```python
from build123d import *

# Parameters (mm, degrees)
BOSS_EXTRUDE1_DEPTH = 5
SKETCH2_R           = 2.1
SKETCH2_R_2         = 1.5
CUT_EXTRUDE1_DEPTH  = 6
SKETCH4_R           = 2.1
CUT_EXTRUDE2_DEPTH  = 6
FILLET1_R           = 2


with BuildPart() as part:
    # Sketch1 → Boss-Extrude1 (new body)
    with BuildSketch(Plane.XY):
        Polygon((-39, 100.232788632), (-12.5, 134.403841263), (-12.5, 167.075), (12.5, 167.075), (12.5, 134.403841263), (39, 100.232788632), (39, 52.075), (27.012855738, 52.075), (-27.012855738, 52.075), (-39, 52.075), align=None)
    extrude(amount=BOSS_EXTRUDE1_DEPTH)

    # Sketch2 → Cut-Extrude1 (cut, through all)
    with BuildSketch(Plane(origin=(0, 0, 0), x_dir=(-1, 0, 0), z_dir=(0, 0, -1))):
        with Locations((-32, 92.575)):
            Circle(SKETCH2_R)
        with Locations((32, 92.575)):
            Circle(SKETCH2_R)
        with Locations((8, 162.075)):
            Circle(SKETCH2_R)
        with Locations((-8, 162.075)):
            Circle(SKETCH2_R)
        with Locations((-18, 112.575)):
            Circle(SKETCH2_R_2)
    extrude(amount=-CUT_EXTRUDE1_DEPTH, mode=Mode.SUBTRACT)

    # Sketch4 → Cut-Extrude2 (cut, through all)
    with BuildSketch(Plane(origin=(0, 0, 0), x_dir=(-1, 0, 0), z_dir=(0, 0, -1))):
        with Locations((-32, 60.075)):
            Circle(SKETCH4_R)
        with Locations((32, 60.075)):
            Circle(SKETCH4_R)
        with Locations((0, 60.075)):
            Circle(SKETCH4_R)
        with Locations((0, 112.575)):
            Circle(SKETCH4_R)
        with Locations((0, 92.575)):
            Circle(SKETCH4_R)
    extrude(amount=-CUT_EXTRUDE2_DEPTH, mode=Mode.SUBTRACT)

    # Fillet1
    fillet1_edges = [part.edges().sort_by_distance(p)[0] for p in [
        (-39, 100.232788632, 2.5),
        (-12.5, 167.075, 2.5),
        (12.5, 167.075, 2.5),
        (39, 100.232788632, 2.5),
        (39, 52.075, 2.5),
        (-39, 52.075, 2.5),
    ]]
    fillet(fillet1_edges, radius=FILLET1_R)


solid = part.part
```
Could you check a few things on this model? Use its own coordinates, in mm. A direction names the side the tool comes from. Round coordinates to 2 decimals unless told otherwise and drop trailing zeros. Write each loop counter-clockwise with the first axis right and the second up, starting at its lowest first coordinate (ties: lowest second). Pieces come first, ordered by that corner, then holes.
(1) Thinking about a two-plate mould opening in Y: for faces 3 (the face through (1, 98, 5)), 4 (the face through (-1, 52.075, 2)), 5 (the face through (0.455, 110.525, 2.465)), which applies, +Y half, -Y half, draft (parallel to the pull), parting line (faces both ways), or undercut?
Findings below:
face 3: draft
face 4: -Y half
face 5: undercut
(2) If I drill on probe 1 along Y at (x, z) = (-32, 3.2) (3 decimals); probe 2 along Y at (x, z) = (0, 1.7) (3 decimals); probe 3 along X at (y, z) = (61.5, 0.25), over which ranges is the centre line in solid material (lowest first)?
Findings below:
probe 1: y = 52.075 to 57.975, 62.175 to 90.475, 94.675 to 109.259
probe 2: y = 52.075 to 57.975, 62.175 to 90.475, 94.675 to 110.475, 114.675 to 167.075
probe 3: x = -39 to -33.54, -30.46 to -1.54, 1.54 to 30.46, 33.54 to 39
(3) Suppose I cut it at D-D on z = 2.95. State how many separate pieces and enclosed holes the cut face has, and give its area (3 significant figures).
Findings below:
separate pieces: 1
enclosed holes: 10
area: 6,200 mm2
(4) Suppose I cut it at A-A on x = 0. Write out the boundary of the cut face in (y, z) (3 decimals), and give its area (3 significant figures).
Findings below:
outline: (52.075, 0) - (57.975, 0) - (57.975, 5) - (52.075, 5) - close; (62.175, 0) - (90.475, 0) - (90.475, 5) - (62.175, 5) - close; (94.675, 0) - (110.475, 0) - (110.475, 5) - (94.675, 5) - close; (114.675, 0) - (167.075, 0) - (167.075, 5) - (114.675, 5) - close
area: 512 mm2
(5) Suppose I cut it at B-B on x = 8. Write out the boundary of the cut face in (y, z) (3 decimals).
Findings below:
outline: (52.075, 0) - (159.975, 0) - (159.975, 5) - (52.075, 5) - close; (164.175, 0) - (167.075, 0) - (167.075, 5) - (164.175, 5) - close
(6) Which directions (+Z, -Z, +X, -X, +Y, -Y) give clear straight access to the entire face, cutting with the end or side of a thin tool? Please do faces 1 (the face through (8.455, 160.025, 2.465)), 2 (the face through (12.5, 150, 2)).
Findings below:
face 1: +Z, -Z
face 2: +Z, -Z, +X, +Y
(7) For pin 1 (4 mm diameter, centred on x = 0, y = 92.575, fed in from +Z), with a flat end and sliding along its axis, tell me the tip position at first contact or that it passes through.
Findings below:
pin 1: passes through
(8) Suppose I cut it at C-C on x = -32. Write out the boundary of the cut face in (y, z) (3 decimals), and give its area (3 significant figures).
Findings below:
outline: (52.075, 0) - (57.975, 0) - (57.975, 5) - (52.075, 5) - close; (62.175, 0) - (90.475, 0) - (90.475, 5) - (62.175, 5) - close; (94.675, 0) - (109.259, 0) - (109.259, 5) - (94.675, 5) - close
area: 244 mm2
